Check sheet for the modelled part. Datum: model origin and axes. Units: mm. A direction names the side the tool comes from. Round coordinates to 2 decimals unless told otherwise and drop trailing zeros.
Item 1: Release check for a two-part mould opening along X. For faces 1 (the cylindrical face through (28.14, 8.86, 13.99)), 2 (the flat face through (-27, 22, 8)), 3 (the cylindrical face through (2.41, 36.42, 12.44)) record: +X half, -X half, draft (parallel to the pull), parting line (faces both ways), or undercut.
Item 2: Tool access check on faces 4 (the cylindrical face through (-5.5, -24.9, 11.5)), 5 (the flat face through (1, -1, 17)). Record the directions out of +Z, -Z, +X, -X, +Y, -Y that give a thin tool (end or side, any length) a straight path to the whole face; none if there is none.
Item 3: Go/stop test with flat-tipped pins: pin 1 Ø5 at (y, z) = (-27, 14) entering from -X; pin 2 Ø1.5 at (y, z) = (-16, 10) entering from -X; pin 3 Ø1.5 at (y, z) = (23.5, 12.5) entering from -X; pin 4 Ø1 at (x, y) = (-25, 28.5) entering from +Z. Record where each tip stops, or that it passes through.
Item 4: Material ranges on line 1 (Y direction, x = 0, z = 14.55); line 2 (X direction, y = 5, z = 11) (3 decimals), recorded low to high.
from build123d import *

# Parameters (mm, degrees)
SKETCH_1_R          = 25.5
SKETCH_1_R_2        = 23.5
EXTRUDE_2_DEPTH     = 15
SKETCH_3_R          = 36.5
SKETCH_3_R_2        = 29.5
EXTRUDE_3_DEPTH     = 15
SKETCH_6_R          = 47.852289075
CUT_EXTRUDE_1_DEPTH = 8
SKETCH_9_R          = 36.5
EXTRUDE_5_DEPTH     = 2


with BuildPart() as part:
    # Sketch 1 → Extrude 2 (new body)
    with BuildSketch(Plane.XY):
        Circle(SKETCH_1_R)
        Circle(SKETCH_1_R_2, mode=Mode.SUBTRACT)
    extrude(amount=EXTRUDE_2_DEPTH)


with BuildPart() as body_2:
    # Sketch 3 → Extrude 3 (new body)
    with BuildSketch(Plane.XY):
        Circle(SKETCH_3_R)
        Circle(SKETCH_3_R_2, mode=Mode.SUBTRACT)
    extrude(amount=EXTRUDE_3_DEPTH)

    # Sketch 5 → Cut-Revolve 2 (revolve, cut)
    with BuildSketch(Plane(origin=(0, 0, 0), x_dir=(1, 0, 0), z_dir=(0, 1, 0))):
        with BuildLine():
            Line((-29.5, -3), (-29.5, -13))
            ThreePointArc((-29.5, -13), (-34.5, -8), (-29.5, -3))
        make_face()
    revolve(axis=Axis((0, 0, 0), (0, 0, 1)), mode=Mode.SUBTRACT)


with BuildPart() as cut_extrude_1_tool:
    # Sketch 6 → Cut-Extrude 1 (new body)
    with BuildSketch(Plane(origin=(0, 0, 0), x_dir=(-1, 0, 0), z_dir=(0, 0, -1))):
        Circle(SKETCH_6_R)
    extrude(amount=-CUT_EXTRUDE_1_DEPTH)


with BuildPart() as part_1:
    add(part.part)

    # Cut-Extrude 1: cut by cut_extrude_1_tool
    add(cut_extrude_1_tool.part, mode=Mode.SUBTRACT)



with BuildPart() as body_2_1:
    add(body_2.part)

    # Cut-Extrude 1: cut by cut_extrude_1_tool
    add(cut_extrude_1_tool.part, mode=Mode.SUBTRACT)


with BuildPart() as part_2:
    add(part_1.part)

    add(body_2_1.part)  # Extrude 5 merges body 2
    # Sketch 9 → Extrude 5 (add)
    with BuildSketch(Plane.XY.offset(15)):
        with Locations(Location((0, 0, 0), (0, 0, 180))):
            Circle(SKETCH_9_R)
    extrude(amount=EXTRUDE_5_DEPTH)


solid = part_2.part
Response values:
1. face 1: undercut
1. face 2: draft
1. face 3: parting line
2. face 4: -Z
2. face 5: +Z, +X, -X, +Y, -Y
3. pin 1: stops at x = -27.06
3. pin 2: stops at x = -33.16
3. pin 3: stops at x = -28.54
3. pin 4: passes through
4. line 1: y = -36.5 to -29.5, -25.5 to -23.5, 23.5 to 25.5, 29.5 to 36.5
4. line 2: x = -36.156 to -33.125, -25.005 to -22.962, 22.962 to 25.005, 33.125 to 36.156
